Design review of the part built by this model. Coordinates are the model's own, in mm. A direction names the side the tool comes from. Round coordinates to 2 decimals unless told otherwise and drop trailing zeros. Order: outer loops, then holes, each group sorted by start corner. A loop starts at its lowest first (then second) coordinate and runs counter-clockwise, first axis right, second up. Notation, with made-up numbers: M -38,-14.75 L -32,-14.75 A8 cw -32,-1.75 Z; hole C 70.25,50.25 d11. An arc over 180 degrees is marked long. Use a Markdown table: item, result. Add a question column.
(1) Take a section at D-D (x = 57). Write out the cut boundary in (y, z).
(2) Take a section at A-A (x = 9). Write out the cut boundary in (y, z), then the cut area to 3 significant figures.
(3) Machinability: for faces 4 (the face through (80, 40, 2)), 5 (the face through (48.85, -36.91, 2.46)), which of the approach directions +Z, -Z, +X, -X, +Y, -Y give a long, thin tool a straight path to every point of the face, cutting with its end or side? Answer none if there is none.
(4) Take a section at C-C (y = 15). Write out the cut boundary in (x, z), then the cut area to 4 significant figures.
(5) Take a section at B-B (z = 3.45). Count the separate pieces of the cut face and the enclosed holes in it, then the cut area to 3 significant figures.
(6) To check wall thickness, follow probe 1 along Y at (x, z) = (31, 0.2); probe 2 along X at (y, z) = (-6, 4.05); probe 3 along Y at (x, z) = (72.5, 2.1). State the ranges of each line that lie inside material, in increasing order. Write a range as from..to.
(7) The part is to be moulded in two halves that separate along X. For faces 1 (the face through (8.46, 6.56, 2.46)), 2 (the face through (21, 0, 2)), 3 (the face through (1, 2, 3)), say which applies: released by +X, released by -X, zero draft, split by the parting line, or undercut.
(8) For pin 1 (3 mm diameter, centred on x = 30.87, y = 65, fed in from +Z); pin 2 (1.5 mm diameter, centred on y = -18.5, z = 2.5, fed in from -X); pin 3 (2.5 mm diameter, centred on y = 23, z = 2.5, fed in from +X), all flat-tipped, find the tip position at first contact; note any pin that passes through.
```python
from build123d import *

# Parameters (mm, degrees)
SKETCH1_R           = 2.5
SKETCH1_R_2         = 1.5
SKETCH1_R_3         = 11
SKETCH1_R_4         = 1.65
BOSS_EXTRUDE1_DEPTH = 5
FILLET1_R           = 5


with BuildPart() as part:
    # Sketch1 → Boss-Extrude1 (new body)
    with BuildSketch(Plane.XY):
        Polygon((0, 0), (0, 80), (80, 80), (80, 0), (90.043707679, 0), (90.043707679, -45), (41.043707679, -45), (41.043707679, 0), align=None)
        with Locations((9, 71)):
            Circle(SKETCH1_R, mode=Mode.SUBTRACT)
        with Locations((71, 71)):
            Circle(SKETCH1_R, mode=Mode.SUBTRACT)
        with Locations((71, 9)):
            Circle(SKETCH1_R, mode=Mode.SUBTRACT)
        with Locations((9, 9)):
            Circle(SKETCH1_R, mode=Mode.SUBTRACT)
        with Locations((50.043707679, -5)):
            Circle(SKETCH1_R_2, mode=Mode.SUBTRACT)
        with Locations((81.043707679, -5)):
            Circle(SKETCH1_R_2, mode=Mode.SUBTRACT)
        with Locations((50.043707679, -36)):
            Circle(SKETCH1_R_2, mode=Mode.SUBTRACT)
        with Locations((81.043707679, -36)):
            Circle(SKETCH1_R_2, mode=Mode.SUBTRACT)
        with Locations((65.543707679, -20.5)):
            Circle(SKETCH1_R_3, mode=Mode.SUBTRACT)
        with Locations((30.868801214, 15)):
            Circle(SKETCH1_R_4, mode=Mode.SUBTRACT)
        with Locations((30.868801214, 65)):
            Circle(SKETCH1_R_4, mode=Mode.SUBTRACT)
    extrude(amount=BOSS_EXTRUDE1_DEPTH)

    # Fillet1
    fillet1_edges = [part.edges().sort_by_distance(p)[0] for p in [
        (0, 0, 2.5),
        (0, 80, 2.5),
        (80, 80, 2.5),
        (80, 0, 2.5),
        (90.043707679, 0, 2.5),
        (90.043707679, -45, 2.5),
        (41.043707679, -45, 2.5),
        (41.043707679, 0, 2.5),
    ]]
    fillet(fillet1_edges, radius=FILLET1_R)


solid = part.part
```
Verdict:
| question | item | result |
|---|---|---|
| 1 | outline | M -45,0 L -27.43,0 L -27.43,5 L -45,5 Z; M -13.57,0 L 80,0 L 80,5 L -13.57,5 Z |
| 2 | outline | M 0,0 L 6.5,0 L 6.5,5 L 0,5 Z; M 11.5,0 L 68.5,0 L 68.5,5 L 11.5,5 Z; M 73.5,0 L 80,0 L 80,5 L 73.5,5 Z |
| 2 | area | 350 mm^2 |
| 3 | face 4 | +Z, -Z, +X, +Y |
| 3 | face 5 | +Z, -Z |
| 4 | outline | M 0,0 L 29.22,0 L 29.22,5 L 0,5 Z; M 32.52,0 L 80,0 L 80,5 L 32.52,5 Z |
| 4 | area | 383.5 mm^2 |
| 5 | separate pieces | 1 |
| 5 | enclosed holes | 11 |
| 5 | area | 8,080 mm^2 |
| 6 | probe 1 | y = 0..13.36, 16.64..63.36, 66.64..80 |
| 6 | probe 2 | x = 41.04..48.93, 51.16..79.93, 82.16..90.04 |
| 6 | probe 3 | y = -45..-29.02, -11.98..7, 11..69, 73..80 |
| 7 | face 1 | undercut |
| 7 | face 2 | zero draft |
| 7 | face 3 | released by -X |
| 8 | pin 1 | passes through |
| 8 | pin 2 | stops at x = 41.04 |
| 8 | pin 3 | stops at x = 80 |
